Autodesk Fusion 360 part; units mm, degrees
sketch "Skizze1" plane through (0, 0, 0) normal (1, 0, 0) x (0, 0, -1)
  line L0 (0, 0) -> (-16, 0)
  line L1 (-16, 0) -> (-16, 13)
  line L2 (-16, 13) -> (-13, 18)
  line L3 (-13, 18) -> (0, 18)
  line L4 (0, 18) -> (0, 0)
  dimension "d1" = 18
  dimension "d2" = 13
  dimension "d3" = 16
  dimension "d5" = 3
extrude "Extrusion1" add sketch "Skizze1" along normal mid plane 16
fillet "Abrundung5" radius 3 2 edges at (8, 18, 6.5) (-8, 18, 6.5)
fillet "Abrundung1" radius 4 1 edges at (0, 13, 16)
fillet "Abrundung2" radius 2 1 edges at (0, 18, 13)
sketch "Skizze2" plane through (0, 18, 0) normal (0, 1, 0) x (-1, 0, 0)
  line L0 (5, 11.8676) -> (-5, 11.8676)
  line L1 (-5, 0) -> (5, 0)
  circle A0 centre (0, 7) radius 1.5
  circle A1 centre (0, 7) radius 3.5
  line L2 (-5, 11.8676) -> (-5, 0)
  line L3 (5, 0) -> (5, 11.8676)
  dimension "d12" = 3
  dimension "d13" = 7
  dimension "d14" = 7
extrude "Extrusion2" cut sketch "Skizze2" against normal blind 23 contours A0
extrude "Extrusion3" cut sketch "Skizze2" against normal blind 5 contours A1
chamfer "Fase2" distance 2 angle 45 1 edges at (1.3985, 13, 6.4576)
fillet "Abrundung3" radius 1 1 edges at (3.2631, 18, 8.2657)
fillet "Abrundung4" radius 2 1 edges at (0, 18, 0)
Verification items for the finished model (mm, model axes). Round coordinates to 2 decimals unless told otherwise and drop trailing zeros. Order: outer loops, then holes, each group sorted by start corner. A loop starts at its lowest first (then second) coordinate and runs counter-clockwise, first axis right, second up. Notation, with made-up numbers: (47.5, 37.5) - (62.5, 37.5) arc R15 ccw to (62.5, 63.5) - close; hole circle Ø3 at (12.5, 32.5). An arc over 180 degrees is marked (long way). Use CSV: the item, a comma, the result in double quotes.
(1) Mould release check, pull along X, two halves, no side actions. Record for faces 1 (the face through (-7.4, 7.6, 0.57)), 2 (the face through (0.759, 15.028, 3.583)), 3 (the face through (7.4, 7.4, 0.57)): released by +X, released by -X, zero draft, split by the parting line, or undercut.
Entries:
face 1,"released by -X"
face 2,"undercut"
face 3,"released by +X"
(2) Section check D-D on x = -4.75. Record the boundary of the cut face in (y, z), and give its area (3 significant figures).
Entries:
outline,"(0, 0) - (16, 0) arc R2 ccw to (18, 2) - (18, 11.87) arc R2 ccw to (17.03, 13.58) - (13.95, 15.43) arc R4 ccw to (11.89, 16) - (0, 16) - close"
area,"279 mm^2"
(3) Gauge pin test, flat ends, axial feed: pin 1 Ø4 at (x, z) = (0, 7) entering from +Y; pin 2 Ø5.5 at (x, z) = (-1.5, 7.5) entering from +Y; pin 3 Ø3.5 at (x, z) = (0, 7) entering from -Y. Record the tip position at first contact, or that the pin passes through.
Entries:
pin 1,"y = 11.5"
pin 2,"y = 17.99"
pin 3,"y = 0"
(4) Section check C-C on y = 10. Record the boundary of the cut face in (x, z).
Entries:
outline,"(-8, 2) arc R2 ccw to (-6, 0) - (6, 0) arc R2 ccw to (8, 2) - (8, 14) arc R2 ccw to (6, 16) - (-6, 16) arc R2 ccw to (-8, 14) - close; hole circle Ø3 at (0, 7)"
(5) Thickness scan on probe 1 along Z at (x, y) = (0, 4.25); probe 2 along Z at (x, y) = (-1.25, 15); probe 3 along Y at (x, z) = (-0.25, 8.75). Record the ranges inside material, lowest first. Write a range as from..to.
Entries:
probe 1,"0..5.5, 8.5..16"
probe 2,"0..3.73, 10.27..14.8"
probe 3,"0..11.27"
